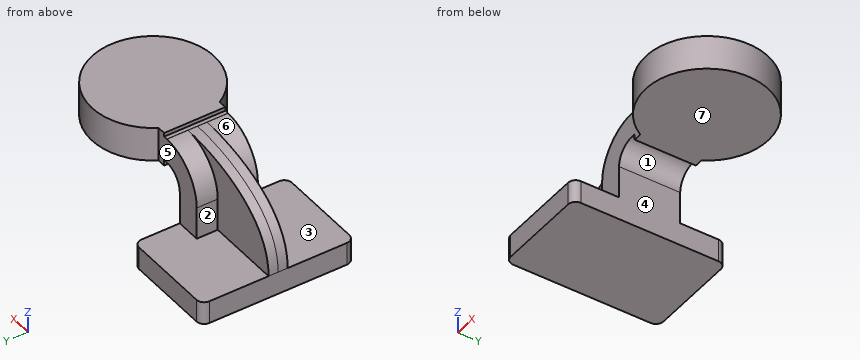
from build123d import *

# Parameters (mm, degrees)
F1_DEPTH = 63.5
F2_DEPTH = 25.4
F3_DEPTH = 7.9375
F5_R     = 6.35


with BuildPart() as f1:
    # F0 (on Front) → F1 (new body, symmetric)
    with BuildSketch(Plane.XZ):
        Polygon((41.275, -9.525), (41.275, 9.525), (20.660926, 9.525), (-41.275, 9.525), (-41.275, -9.525), align=None)
    extrude(amount=F1_DEPTH, both=True)

    # F0 (on Front) → F2 (join, symmetric)
    with BuildSketch(Plane.XZ):
        with BuildLine():
            Line((20.660926, 9.525), (41.275, 9.525))
            Line((41.275, 9.525), (41.275, 36.5252))
            ThreePointArc((41.275, 36.5252), (45.92468, 47.75052), (57.15, 52.4002))
            Line((57.15, 52.4002), (60.325, 52.4002))
            Line((60.325, 52.4002), (60.325, 73.014274))
            Line((60.325, 73.014274), (57.15, 73.014274))
            add(Edge.make_bspline(
                [(56.793396, 73.012532), (56.912382, 73.013238), (57.03125, 73.013819), (57.15, 73.014274)],
                knots=[116.793783, 116.793783, 116.793783, 116.793783, 117.12544, 117.12544, 117.12544, 117.12544], degree=3))
            ThreePointArc((56.793396, 73.012532), (31.222556, 62.200484), (20.660926, 36.5252))
            Line((20.660926, 36.5252), (20.660926, 9.525))
        make_face()
        Polygon((60.325, 73.014274), (60.325, 52.4002), (60.325, 47.625), (111.125, 47.625), (111.125, 76.2), (60.325, 76.2), align=None)
    extrude(amount=F2_DEPTH, both=True)

    # F0 (on Front) → F3 (join, symmetric)
    with BuildSketch(Plane.XZ):
        with BuildLine():
            Line((-41.275, 9.525), (20.660926, 9.525))
            Line((20.660926, 9.525), (20.660926, 36.5252))
            ThreePointArc((20.660926, 36.5252), (31.222556, 62.200484), (56.793396, 73.012532))
            add(Edge.make_bspline(
                [(-41.275, 9.525), (-41.534558, 56.956479), (14.892301, 72.763843), (56.793396, 73.012532)],
                knots=[0, 0, 0, 0, 116.793783, 116.793783, 116.793783, 116.793783], degree=3))
        make_face()
    extrude(amount=F3_DEPTH, both=True)

    # F0 (on Front) → F4 (revolve)
    with BuildSketch(Plane.XZ):
        Polygon((60.325, 73.014274), (60.325, 52.4002), (60.325, 47.625), (111.125, 47.625), (111.125, 76.2), (60.325, 76.2), align=None)
    revolve(axis=Axis((111.125, 0, 61.9125), (0, 0, -1)))

    # F5
    f5_edges = [f1.edges().sort_by_distance(p)[0] for p in [
        (41.275, -63.5, 0),
        (-41.275, -63.5, 0),
        (41.275, 63.5, 0),
        (-41.275, 63.5, 0),
    ]]
    fillet(f5_edges, radius=F5_R)


solid = f1.part
Part model, mm, in its own coordinate system. Face numbers are marked on the shaded views. A direction names the side the tool comes from. Round coordinates to 2 decimals unless told otherwise and drop trailing zeros. Write each loop counter-clockwise with the first axis right and the second up, starting at its lowest first coordinate (ties: lowest second). Pieces come first, ordered by that corner, then holes. Notation, with made-up numbers: M 34,-1 L 52,-1 A26 ccw 52,19 Z; hole C 41,-19 d9. An arc over 180 degrees is marked long. Return JSON: item names as keys, results as strings. Group by question number.
(1) Saw through at B-B on z = 3. Write the cut outline in (x, y) (3 decimals), then the cut area to 3 significant figures.
(2) Saw through at C-C on y = -55. Write the cut outline in (x, z) (3 decimals).
(3) Which spindle directions (+Z, -Z, +X, -X, +Y, -Y) get a long thin tool onto all of the face, cutting with end or side? Do the marked faces 5, 6 and 7. Say none if no direction does.
(4) Saw through at A-A on y = -41. Write the cut outline in (x, z) (3 decimals), then the cut area to 3 significant figures.
(5) Pin check, flat tips, straight feed: pin 1 Ø12 at (x, z) = (63, 56.5) entering from +Y; pin 2 Ø4 at (y, z) = (1, 51) entering from -X; pin 3 Ø8.5 at (y, z) = (20, 29.5) entering from -X. Stop position of each tip, or through.
(6) Saw through at D-D on x = 124. Write the cut outline in (y, z) (3 decimals).
(7) Drill centre lines: probe 1 along Y at (x, z) = (29, 45.5); probe 2 along Z at (x, y) = (105, 35) (3 decimals); probe 3 along Y at (x, z) = (-23.5, 36). Where is each one in solid material? Low to high.
(8) Two-plate mould, pull along X, no slides. Class the marked faces 1, 2, 3 and 4: +X half, -X half, draft (parallel to the pull), parting line (faces both ways), or undercut.
Returned:
{
 "1": {"outline": "M -41.275,-57.15 A6.35 ccw -34.925,-63.5 L 34.925,-63.5 A6.35 ccw 41.275,-57.15 L 41.275,57.15 A6.35 ccw 34.925,63.5 L -34.925,63.5 A6.35 ccw -41.275,57.15 Z", "area": "10,400 mm²"},
 "2": {"outline": "M -41.275,-9.525 L 41.275,-9.525 L 41.275,9.525 L -41.275,9.525 Z"},
 "3": {"face 5": "+Z, -X, +Y", "face 6": "+Z, -X, -Y", "face 7": "-Z, +X, +Y, -Y"},
 "4": {"outline": "M -41.275,-9.525 L 41.275,-9.525 L 41.275,9.525 L -41.275,9.525 Z; M 81.131,47.625 L 141.119,47.625 L 141.119,76.2 L 81.131,76.2 Z", "area": "3,290 mm²"},
 "5": {"pin 1": "y = 28.39", "pin 2": "x = -23.08", "pin 3": "x = 20.66"},
 "6": {"outline": "M -49.141,47.625 L 49.141,47.625 L 49.141,76.2 L -49.141,76.2 Z"},
 "7": {"probe 1": "-25.4 to 25.4", "probe 2": "47.625 to 76.2", "probe 3": "-7.94 to 7.94"},
 "8": {"face 1": "undercut", "face 2": "-X half", "face 3": "draft", "face 4": "+X half"}
}
